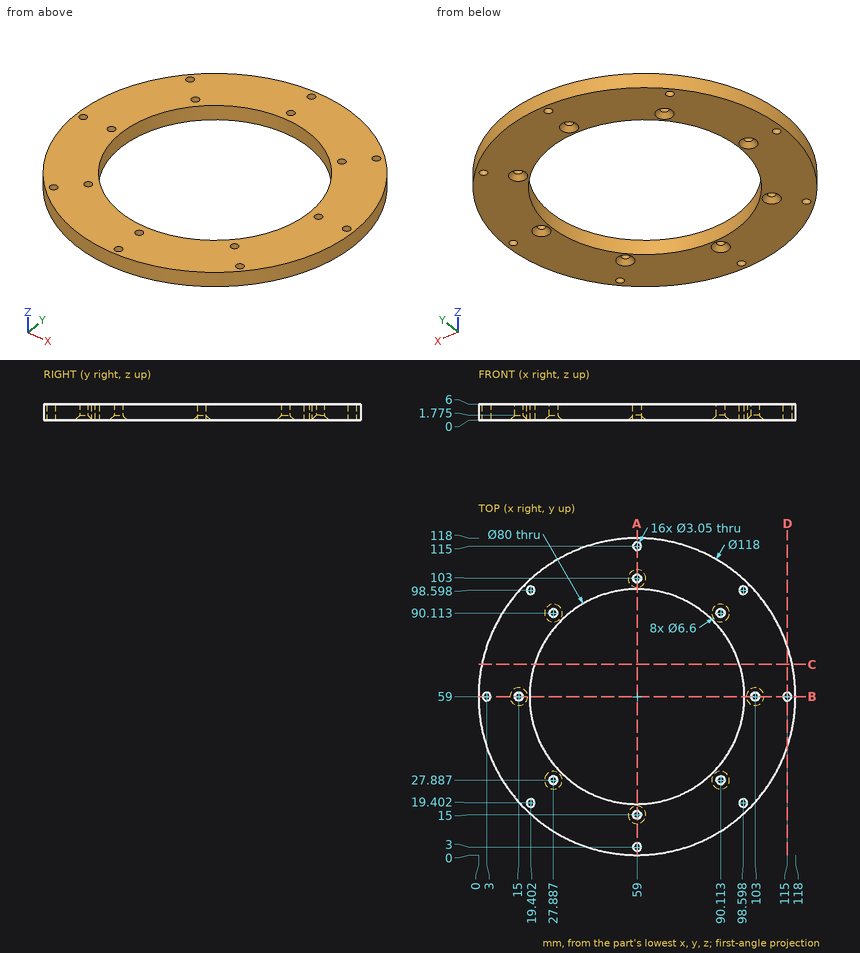
Can you work these out from the drawing? Everything is in mm from the part's minimum corner. Round coordinates to 2 decimals unless told otherwise and drop trailing zeros. Write each loop counter-clockwise with the first axis right and the second up, starting at its lowest first coordinate (ties: lowest second). Pieces come first, ordered by that corner, then holes. Notation, with made-up numbers: (-8, -21.75) - (-3, -21.75) arc R23 cw to (-3, -0.75) - close; hole circle Ø4 at (-34.75, 7.25). An arc over 180 degrees is marked (long way). Put each result on its own line as item: value. Start each with the question number.
(1) I want a section at C-C, the plane y = 71. Please give me the cut outline in (x, z).
(2) I need wall thicknesses on probe 1 along X at (y, z) = (29, 3.35) (1 decimal); probe 2 along Y at (x, z) = (28.5, 3.95) (1 decimal); probe 3 along X at (y, z) = (63, 1). Which ranges of each line are inside material? Lowest first, please.
(3) Will these pins go through, and if not, where does the flat tip stop? pin 1 (1.5 mm diameter, centred on x = 18, z = 1.5, fed in from +Y); pin 2 (3 mm diameter, centred on y = 79.5, z = 3.5, fed in from -X); pin 3 (3 mm diameter, centred on y = 102.5, z = 3.5, fed in from -X).
(4) I want a section at A-A, the plane x = 59. Please give me the cut outline in (y, z) (1 decimal).
(5) I want a section at D-D, the plane x = 115. Please give me the cut outline in (y, z) (1 decimal), plus the area to 3 significant figures.
Here are the results:
1. outline: (1.23, 0) - (20.84, 0) - (20.84, 6) - (1.23, 6) - close; (97.16, 0) - (116.77, 0) - (116.77, 6) - (97.16, 6) - close
2. probe 1: x = 8.2 to 26.8, 28.9 to 32.5, 85.5 to 89.1, 91.2 to 109.8
2. probe 2: y = 8.5 to 26.5, 29.3 to 33.1, 84.9 to 88.7, 91.5 to 109.5
2. probe 3: x = 0.14 to 19.2, 98.8 to 117.86
3. pin 1: stops at y = 102.14
3. pin 2: stops at x = 3.14
3. pin 3: stops at x = 17.56
4. outline: (0, 0) - (1.5, 0) - (1.5, 6) - (0, 6) - close; (4.5, 0) - (11.7, 0) - (13.5, 1.8) - (13.5, 6) - (4.5, 6) - close; (16.5, 1.8) - (18.3, 0) - (19, 0) - (19, 6) - (16.5, 6) - close; (99, 0) - (99.7, 0) - (101.5, 1.8) - (101.5, 6) - (99, 6) - close; (104.5, 1.8) - (106.3, 0) - (113.5, 0) - (113.5, 6) - (104.5, 6) - close; (116.5, 0) - (118, 0) - (118, 6) - (116.5, 6) - close
5. outline: (40.4, 0) - (57.5, 0) - (57.5, 6) - (40.4, 6) - close; (60.5, 0) - (77.6, 0) - (77.6, 6) - (60.5, 6) - close
5. area: 205 mm^2
